```python
from build123d import *

# Parameters (mm, degrees)
SALIENTE_EXTRUIR1_DEPTH = 40
CORTAR_EXTRUIR1_DEPTH   = 110.100828683
CHAFL_N1_SIZE           = 5
CROQUIS3_W              = 52.370156311
CROQUIS3_H              = 5
CORTAR_EXTRUIR2_DEPTH   = 110.100828683
CHAFL_N2_SIZE           = 5
CROQUIS4_W              = 25
CROQUIS4_H              = 25
CORTAR_EXTRUIR3_DEPTH   = 1.2
CROQUIS5_W              = 9
CROQUIS5_H              = 9
CORTAR_EXTRUIR4_DEPTH   = 118.586419677
CROQUIS6_W              = 10
CROQUIS6_H              = 9
CORTAR_EXTRUIR5_DEPTH   = 2
CHAFL_N5_SIZE           = 2
CHAFL_N6_SIZE           = 5


with BuildPart() as part:
    # Croquis1 → Saliente-Extruir1 (new body)
    with BuildSketch(Plane(origin=(0, 0, 0), x_dir=(1, 0, 0), z_dir=(0, 1, 0))):
        Polygon((-0.349963823, 11.66546078), (49.650036177, 11.66546078), (49.650036177, 7.66546078), (21.892676864, 7.66546078), (2.650036177, -11.577179907), (2.650036177, -88.33453922), (-0.349963823, -88.33453922), align=None)
        Polygon((17.650036177, 7.66546078), (2.650036177, -7.33453922), (2.650036177, 7.66546078), align=None, mode=Mode.SUBTRACT)
    extrude(amount=SALIENTE_EXTRUIR1_DEPTH)

    # Croquis2 → Cortar-Extruir1 (cut, through all)
    with BuildSketch(Plane.ZY.offset(0.349963823)):
        with BuildLine():
            Line((58.33453922, 37), (78.33453922, 37))
            ThreePointArc((78.33453922, 37), (80.33453922, 35), (78.33453922, 33))
            Line((78.33453922, 33), (58.33453922, 33))
            ThreePointArc((58.33453922, 33), (56.33453922, 35), (58.33453922, 37))
        make_face()
        with BuildLine():
            Line((58.33453922, 7), (78.33453922, 7))
            ThreePointArc((78.33453922, 7), (80.33453922, 5), (78.33453922, 3))
            Line((78.33453922, 3), (58.33453922, 3))
            ThreePointArc((58.33453922, 3), (56.33453922, 5), (58.33453922, 7))
        make_face()
    extrude(amount=-CORTAR_EXTRUIR1_DEPTH, mode=Mode.SUBTRACT)

    # Chaflán1
    chafl_n1_edges = [part.edges().sort_by_distance(p)[0] for p in [
        (-0.349963823, 20, -11.66546078),
        (2.650036177, 20, -7.66546078),
    ]]
    chamfer(chafl_n1_edges, length=CHAFL_N1_SIZE)

    # Croquis3 → Cortar-Extruir2 (cut, through all)
    with BuildSketch(Plane.ZY.offset(0.349963823)):
        with Locations((14.519617376, 2.5)):
            Rectangle(CROQUIS3_W, CROQUIS3_H)
        with Locations((14.519617376, 37.5)):
            Rectangle(CROQUIS3_W, CROQUIS3_H)
    extrude(amount=-CORTAR_EXTRUIR2_DEPTH, mode=Mode.SUBTRACT)

    # Chaflán2
    chafl_n2_edges = [part.edges().sort_by_distance(p)[0] for p in [
        (1.150036177, 35, 40.704695531),
        (1.150036177, 5, 40.704695531),
    ]]
    chamfer(chafl_n2_edges, length=CHAFL_N2_SIZE - 0.0001)  # a hair under: the kernel refuses the full size

    # Croquis4 → Cortar-Extruir3 (cut)
    with BuildSketch(Plane(origin=(0, 0, -11.66546078), x_dir=(-1, 0, 0), z_dir=(0, 0, -1))):
        with Locations((-34.650036177, 20)):
            Rectangle(CROQUIS4_W, CROQUIS4_H)
    extrude(amount=-CORTAR_EXTRUIR3_DEPTH, mode=Mode.SUBTRACT)

    # Croquis5 → Cortar-Extruir4 (cut, through all)
    with BuildSketch(Plane(origin=(0, 0, -10.46546078), x_dir=(-1, 0, 0), z_dir=(0, 0, -1))):
        with Locations((-32.650036177, 20)):
            Rectangle(CROQUIS5_W, CROQUIS5_H)
    extrude(amount=-CORTAR_EXTRUIR4_DEPTH, mode=Mode.SUBTRACT)

    # Croquis6 → Cortar-Extruir5 (cut)
    with BuildSketch(Plane(origin=(0, 0, -10.46546078), x_dir=(-1, 0, 0), z_dir=(0, 0, -1))):
        with Locations((-42.150036177, 20)):
            Rectangle(CROQUIS6_W, CROQUIS6_H)
    extrude(amount=-CORTAR_EXTRUIR5_DEPTH, mode=Mode.SUBTRACT)

    # Chaflán5
    chafl_n5_edges = [part.edges().sort_by_distance(p)[0] for p in [
        (49.650036177, 5, -9.66546078),
        (49.650036177, 35, -9.66546078),
    ]]
    chamfer(chafl_n5_edges, length=CHAFL_N5_SIZE)

    # Chaflán6
    chafl_n6_edges = [part.edges().sort_by_distance(p)[0] for p in [
        (1.150036177, 40, 88.33453922),
        (1.150036177, 0, 88.33453922),
    ]]
    chamfer(chafl_n6_edges, length=CHAFL_N6_SIZE)


solid = part.part
```
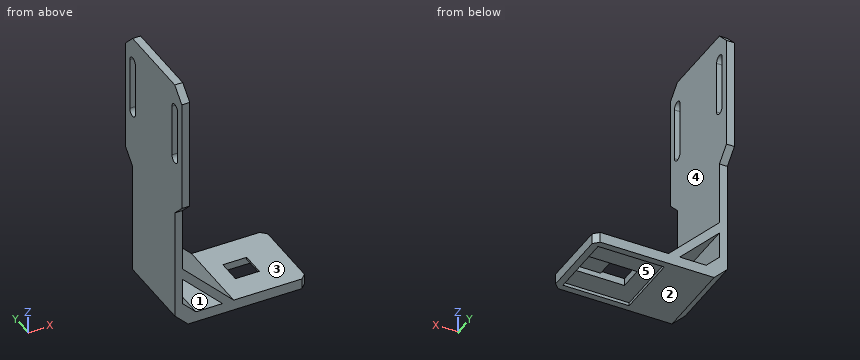
Source: CAD feature listing. Evaluate the final solid. Frame: model axes, mm. Face numbers are marked on the shaded views. A direction names the side the tool comes from. Round coordinates to 2 decimals unless told otherwise and drop trailing zeros. Order: outer loops, then holes, each group sorted by start corner. A loop starts at its lowest first (then second) coordinate and runs counter-clockwise, first axis right, second up. Notation, with made-up numbers: (44, -19.75) -> (87, -19.75) arc R13 cw to (87, -8.75) -> close; hole circle Ø11 at (34, 55). An arc over 180 degrees is marked (long way). One line per item, written item: value. Start each with the question number.
Q1. Section query D-D (x = 44.5). Return the cut outline in (y, z).
Q2. Section query C-C (y = 8.5). Return the cut outline in (x, z).
Q3. Pin query (flat end, axial travel): pin 1 (1 mm diameter, centred on x = 35, z = -11, fed in from +Y); pin 2 (8 mm diameter, centred on x = 14.5, y = 27.5, fed in from +Z); pin 3 (8.5 mm diameter, centred on x = 34, y = 18, fed in from +Z); pin 4 (10 mm diameter, centred on x = 17, z = 7.5, fed in from -Y). Return the tip coordinate at first contact, or that it passes through.
Q4. Access query for the marked faces 1, 2 and 3. Directions: +Z, -Z, +X, -X, +Y, -Y. A direction counts if a zero-diameter tool reaches every point of the face in a straight line with its end or side. Return the directions, or none.
Q5. Draft query along Y for the marked faces 4 and 5. Return one class per face: pulls with the +Y half, pulls with the -Y half, needs draft (parallel to the pull), parting line crosses it, or undercut.
Q6. Section query B-B (z = 65.5). Return the cut outline in (x, y).
Q7. Section query A-A (y = 19). Return the cut outline in (x, z).
Q8. Material intervals for probe 1 along Z at (x, y) = (42, 5.5); probe 2 along X at (y, z) = (9, 21); probe 3 along Z at (x, y) = (12, 13.5), sorted ascending.
Findings below:
1. outline: (5, -11.67) -> (7.5, -11.67) -> (7.5, -10.47) -> (15.5, -10.47) -> (15.5, -8.47) -> (24.5, -8.47) -> (24.5, -10.47) -> (32.5, -10.47) -> (32.5, -11.67) -> (35, -11.67) -> (35, -7.67) -> (5, -7.67) -> close
2. outline: (-0.35, -6.67) -> (4.65, -11.67) -> (22.15, -11.67) -> (22.15, -10.47) -> (47.15, -10.47) -> (47.15, -11.67) -> (49.65, -11.67) -> (49.65, -7.67) -> (21.89, -7.67) -> (2.65, 11.58) -> (2.65, 88.33) -> (-0.35, 88.33) -> close; hole (2.65, -2.67) -> (7.65, -7.67) -> (17.65, -7.67) -> (2.65, 7.33) -> close
3. pin 1: y = 35
3. pin 2: z = 3.73
3. pin 3: z = -7.67
3. pin 4: through
4. face 1: +Y, -Y
4. face 2: -Z, +X, -X, +Y, -Y
4. face 3: +Z, +X, +Y, -Y
5. face 4: needs draft
5. face 5: undercut
6. outline: (-0.35, 0) -> (2.65, 0) -> (2.65, 3) -> (-0.35, 3) -> close; (-0.35, 7) -> (2.65, 7) -> (2.65, 33) -> (-0.35, 33) -> close; (-0.35, 37) -> (2.65, 37) -> (2.65, 40) -> (-0.35, 40) -> close
7. outline: (-0.35, -6.67) -> (4.65, -11.67) -> (22.15, -11.67) -> (22.15, -10.47) -> (28.15, -10.47) -> (28.15, -7.67) -> (21.89, -7.67) -> (2.65, 11.58) -> (2.65, 88.33) -> (-0.35, 88.33) -> close; (37.15, -8.47) -> (47.15, -8.47) -> (47.15, -11.67) -> (49.65, -11.67) -> (49.65, -7.67) -> (37.15, -7.67) -> close; hole (2.65, -2.67) -> (7.65, -7.67) -> (17.65, -7.67) -> (2.65, 7.33) -> close
8. probe 1: -11.67 to -7.67
8. probe 2: -0.35 to 2.65
8. probe 3: -11.67 to -7.67, -2.02 to 2.23
